The model under review builds one solid part; all positions refer to its coordinate system, in mm. A direction names the side the tool comes from. Give positions to 0.01 mm unless a question says otherwise; leave off trailing zeros. Write each loop counter-clockwise with the first axis right and the second up, starting at its lowest first coordinate (ties: lowest second). Pieces come first, ordered by that corner, then holes. Notation, with made-up numbers: M 34.25,61 L 93.25,61 A22 ccw 93.25,91 Z; hole C 35.25,9 d6. An arc over 180 degrees is marked long. Write each question's results on one line, items separated by ' | '. Start each with the question number.
from build123d import *

# Parameters (mm, degrees)
SKETCH2_R           = 10
BOSS_EXTRUDE1_DEPTH = 12.5
SKETCH3_R           = 15
BOSS_EXTRUDE2_DEPTH = 4
SKETCH4_R           = 10
BOSS_EXTRUDE3_DEPTH = 34.3
FILLET1_R           = 1


with BuildPart() as part:
    # Sketch2 → Boss-Extrude1 (new body)
    with BuildSketch(Plane.XY):
        Circle(SKETCH2_R)
    boss_extrude1 = extrude(amount=BOSS_EXTRUDE1_DEPTH)

    # Sketch3 → Boss-Extrude2 (add)
    with BuildSketch(Plane.XY.offset(12.5)):
        Circle(SKETCH3_R)
    boss_extrude2 = extrude(amount=BOSS_EXTRUDE2_DEPTH)

    # Sketch4 → Boss-Extrude3 (add)
    with BuildSketch(Plane.XY.offset(16.5)):
        Circle(SKETCH4_R)
    boss_extrude3 = extrude(amount=BOSS_EXTRUDE3_DEPTH)

    # Mirror1: Boss-Extrude1, Boss-Extrude2, Boss-Extrude3 across plane
    add(boss_extrude1.mirror(Plane.XY))
    add(boss_extrude2.mirror(Plane.XY))
    add(boss_extrude3.mirror(Plane.XY))

    # Fillet1
    fillet1_edges = [part.edges().sort_by_distance(p)[0] for p in [
        (-10, 0, 50.8),
        (-10, 0, -50.8),
    ]]
    fillet(fillet1_edges, radius=FILLET1_R)


solid = part.part
(1) Wall thickness on L1, parallel to Z at x = -10, y = 7; L2, parallel to X at y = -0.25, z = 7; L3, parallel to X at y = -13.5, z = 15: over which ranges is each line inside the solid? List them lowest first.
(2) Clearance check with flat-ended pins moving along their axes: P1, Ø4, axis at y = 6, z = 26.5, coming from the -X side; P2, Ø2, axis at y = -5.5, z = 12, coming from the +X side; P3, Ø1.5, axis at y = 2.5, z = 11.5, coming from the +X side; P4, Ø10, axis at x = 3, z = -12.5, coming from the -Y side. State where each tip first meets the part, or that it passes through.
(3) Add section C-C (z = 6). State the section outline as (x, y) points.
(4) Add section A-A (y = 0). State the section outline as (x, z) points.
(5) Machinability: for faces 1 (the flat face through (0, 0, -50.8)), 2 (the cylindrical face through (-2.17, -9.76, 0.18)), 3 (the cylindrical face through (-2.17, -9.76, -32.92)), 4 (the flat face through (3, -10, 16.5)), 5 (the flat face through (0, 0, 50.8)), which of the approach directions +Z, -Z, +X, -X, +Y, -Y give a long, thin tool a straight path to every point of the face, cutting with its end or side? Answer none if there is none.
Calculated:
1) L1: z = -16.5 to -12.5, 12.5 to 16.5 | L2: x = -10 to 10 | L3: x = -6.54 to 6.54
2) P1: stops at x = -9.17 | P2: stops at x = 14.27 | P3: stops at x = 9.85 | P4: stops at y = -15
3) outline: C 0,0 d20
4) outline: M -15,-16.5 L -10,-16.5 L -10,-49.8 A1 ccw -9,-50.8 L 9,-50.8 A1 ccw 10,-49.8 L 10,-16.5 L 15,-16.5 L 15,-12.5 L 10,-12.5 L 10,12.5 L 15,12.5 L 15,16.5 L 10,16.5 L 10,49.8 A1 ccw 9,50.8 L -9,50.8 A1 ccw -10,49.8 L -10,16.5 L -15,16.5 L -15,12.5 L -10,12.5 L -10,-12.5 L -15,-12.5 Z
5) face 1: -Z, +X, -X, +Y, -Y | face 2: none | face 3: -Z | face 4: +Z | face 5: +Z, +X, -X, +Y, -Y
